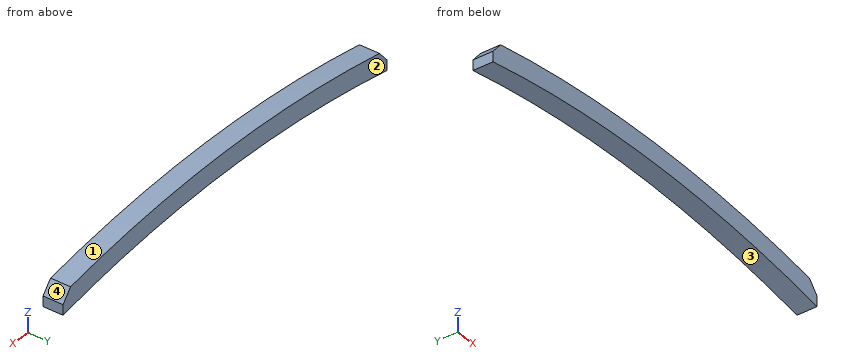
from build123d import *

# Parameters (mm, degrees)
F1_DEPTH    = 19.05
F2_T1_DEPTH = 68.6123794065


# Not quite as in the source:
# - a fillet or chamfer that OpenCascade refuses, or shapes differently, is made with other operations: its cross-section is extruded or revolved along the edge and cut away or added


with BuildPart() as f1:
    # F0 (on Front) → F1 (new body)
    with BuildSketch(Plane.XZ):
        with BuildLine():
            ThreePointArc((-203.2046722501, -19.05), (0, 0), (203.2046722501, -19.05))
            Line((203.2046722501, -19.05), (203.2046722501, 0.3318805247))
            ThreePointArc((203.2046722501, 0.3318805247), (0, 19.0500002354), (-203.2046722501, 0.3318805247))
            Line((-203.2046722501, 0.3318805247), (-203.2046722501, -19.05))
        make_face()
    extrude(amount=F1_DEPTH)

    # F2: chamfer of 9.525 on 2 edges, made by hand

    # F2_s2 → F2_t1 (cut)
    with BuildSketch(Plane.XZ.offset(-24.7811897032)):
        with BuildLine():
            Line((-193.4976640556, 2.339657905), (-203.4494965837, -9.5268916064))
            Line((-203.4494965837, -9.5268916064), (-203.6399965837, -9.5268916064))
            ThreePointArc((-203.6399965837, -9.5268916064), (-203.3951722501, -4.5975055408), (-203.3951722501, 0.3318805247))
            Line((-203.3951722501, 0.3318805247), (-203.2394726328, 0.5191749009))
            ThreePointArc((-203.2394726328, 0.5191749009), (-198.3652719444, 1.4136040473), (-193.5308439656, 2.5272461338))
            Line((-193.5308439656, 2.5272461338), (-193.4976640556, 2.339657905))
        make_face()
        with BuildLine():
            Line((193.4976640556, 2.339657905), (203.4494965837, -9.5268916064))
            Line((203.4494965837, -9.5268916064), (203.6399965837, -9.5268916064))
            ThreePointArc((203.6399965837, -9.5268916064), (203.3951722501, -4.5975055408), (203.3951722501, 0.3318805247))
            Line((203.3951722501, 0.3318805247), (203.2394726328, 0.5191749009))
            ThreePointArc((203.2394726328, 0.5191749009), (198.3652719444, 1.4136040473), (193.5308439656, 2.5272461338))
            Line((193.5308439656, 2.5272461338), (193.4976640556, 2.339657905))
        make_face()
    extrude(amount=F2_T1_DEPTH, mode=Mode.SUBTRACT)


solid = f1.part
Here's how the part is built. I have some questions about the finished solid (model axes, mm). Face numbers are marked on the shaded views. Round coordinates to 2 decimals unless told otherwise and drop trailing zeros. Loops run counter-clockwise (first coordinate to the right, second up) from the corner with the lowest first, then second, coordinate; pieces in that order, holes last.
1. If I drill on line 1 along X through (y, z) = (-6, 1); line 2 along Z through (x, y) = (-141.5, -9.25); line 3 along Z through (x, y) = (176.5, -2.25), over which ranges is the centre line in solid material (lowest first)?
Answer list:
line 1: x = -194.62 to 194.62
line 2: z = -9.2 to 10.01
line 3: z = -14.34 to 4.96
2. If we section it at C-C on x = 105: Write out the boundary of the cut face in (y, z), plus the area to 3 significant figures.
Answer list:
outline: (-19.05, -5.05) - (0, -5.05) - (0, 14.08) - (-19.05, 14.08) - close
area: 365 mm2
3. If we section it at A-A on z = -13: Write out the boundary of the cut face in (x, y), plus the area to 3 significant figures.
Answer list:
outline: (-203.2, -19.05) - (-168.1, -19.05) - (-168.1, 0) - (-203.2, 0) - close; (168.1, -19.05) - (203.2, -19.05) - (203.2, 0) - (168.1, 0) - close
area: 1,340 mm2
4. If we section it at B-B on y = -11.5: Write out the boundary of the cut face in (x, z), plus the area to 3 significant figures.
Answer list:
outline: (-203.2, -19.05) arc R1093.31 cw to (203.2, -19.05) - (203.2, -9.23) - (193.74, 2.05) arc R1112.36 ccw to (-193.74, 2.05) - (-203.2, -9.23) - close
area: 7,700 mm2
5. For P1, Ø2, axis at y = -15, z = -2, coming from the +X side; P2, Ø5, axis at x = 84, y = -12, coming from the +Z side, each with a flat end and sliding along its axis, tell me the tip position at first contact or that it passes through.
Answer list:
P1: stops at x = 197.98
P2: stops at z = 16.06
6. We'd pull the mould along X, two halves only. Please class the marked faces 1, 2, 3 and 4: +X half, -X half, draft (parallel to the pull), parting line (faces both ways), or undercut.
Answer list:
face 1: parting line
face 2: draft
face 3: undercut
face 4: +X half
